from build123d import *

# Parameters (mm, degrees)
SKETCH1_W           = 57
SKETCH1_H           = 57
BOSS_EXTRUDE1_DEPTH = 113
SKETCH2_R           = 11
CUT_EXTRUDE1_DEPTH  = 103
SKETCH3_R           = 2.55
CUT_EXTRUDE2_DEPTH  = 120.97291361
FILLET2_R           = 3
SKETCH4_R           = 19
BOSS_EXTRUDE2_DEPTH = 1.6
FILLET4_R           = 3
SKETCH6_R           = 4
BOSS_EXTRUDE3_DEPTH = 24
SKETCH7_R           = 6
BOSS_EXTRUDE4_DEPTH = 2
CIRPATTERN4_COUNT   = 4
FILLET5_R           = 4
FILLET6_R           = 4


with BuildPart() as part:
    # Sketch1 → Boss-Extrude1 (new body)
    with BuildSketch(Plane.XY):
        Rectangle(SKETCH1_W, SKETCH1_H)
    extrude(amount=BOSS_EXTRUDE1_DEPTH)

    # Sketch2 → Cut-Extrude1 (cut)
    with BuildSketch(Plane(origin=(0, 0, 0), x_dir=(-1, 0, 0), z_dir=(0, 0, -1))):
        with Locations((-28.5, 28.5)):
            Circle(SKETCH2_R)
    cut_extrude1 = extrude(amount=-CUT_EXTRUDE1_DEPTH, mode=Mode.SUBTRACT)

    # Sketch3 → Cut-Extrude2 (cut, through all)
    with BuildSketch(Plane.XY.offset(113)):
        with Locations((-23.5, 23.5)):
            Circle(SKETCH3_R)
        with Locations((23.5, 23.5)):
            Circle(SKETCH3_R)
        with Locations((23.5, -23.5)):
            Circle(SKETCH3_R)
        with Locations((-23.5, -23.5)):
            Circle(SKETCH3_R)
    extrude(amount=-CUT_EXTRUDE2_DEPTH, mode=Mode.SUBTRACT)

    # Fillet2
    fillet2_edges = [part.edges().sort_by_distance(p)[0] for p in [
        (28.5, 28.5, 108),
    ]]
    fillet(fillet2_edges, radius=FILLET2_R)

    # Sketch4 → Boss-Extrude2 (add)
    with BuildSketch(Plane.XY.offset(113)):
        Circle(SKETCH4_R)
    extrude(amount=BOSS_EXTRUDE2_DEPTH)

    # Fillet4
    fillet4_edges = [part.edges().sort_by_distance(p)[0] for p in [
        (-28.5, 28.5, 56.5),
        (28.5, -28.5, 56.5),
        (-28.5, -28.5, 56.5),
    ]]
    fillet(fillet4_edges, radius=FILLET4_R)

    # Sketch6 → Boss-Extrude3 (add)
    with BuildSketch(Plane.XY.offset(114.6)):
        Circle(SKETCH6_R)
    extrude(amount=BOSS_EXTRUDE3_DEPTH)

    # Sketch7 → Boss-Extrude4 (add)
    with BuildSketch(Plane.ZY.offset(28.5)):
        with Locations(Location((12.240016964, 0, 0), (0, 0, 90))):
            Circle(SKETCH7_R)
    extrude(amount=BOSS_EXTRUDE4_DEPTH)

    # CirPattern4: Cut-Extrude1 ×4 about axis
    cirpattern4_axis = Axis((0, 0, 0), (0, 0, 1))
    for i in range(1, CIRPATTERN4_COUNT):
        add(cut_extrude1.rotate(cirpattern4_axis, i * 360 / CIRPATTERN4_COUNT), mode=Mode.SUBTRACT)

    # Fillet5
    fillet5_edges = [part.edges().sort_by_distance(p)[0] for p in [
        (-28.5, -17.5, 51.5),
        (-17.5, -28.5, 51.5),
        (17.5, -28.5, 51.5),
        (28.5, -17.5, 51.5),
        (28.5, 17.5, 51.5),
        (17.5, 28.5, 51.5),
        (-28.5, 17.5, 51.5),
        (-17.5, 28.5, 51.5),
    ]]
    fillet(fillet5_edges, radius=FILLET5_R)

    # Fillet6
    fillet6_edges = [part.edges().sort_by_distance(p)[0] for p in [
        (-28.5, 0, 0),
        (-20.721825407, 20.721825407, 0),
        (0, 28.5, 0),
        (20.721825407, 20.721825407, 0),
        (28.5, 0, 0),
        (20.721825407, -20.721825407, 0),
        (0, -28.5, 0),
        (-20.721825407, -20.721825407, 0),
        (27.683289703, -16.465287988, 0),
        (16.465287988, -27.683289703, 0),
        (-16.465287988, -27.683289703, 0),
        (-27.683289703, -16.465287988, 0),
        (27.683289703, 16.465287988, 0),
        (16.465287988, 27.683289703, 0),
        (-16.465287988, 27.683289703, 0),
        (-27.683289703, 16.465287988, 0),
    ]]
    fillet(fillet6_edges, radius=FILLET6_R)


solid = part.part
CAD build for the part. Positions are in the model's coordinates, mm. A direction names the side the tool comes from. Round coordinates to 2 decimals unless told otherwise and drop trailing zeros. Write each loop counter-clockwise with the first axis right and the second up, starting at its lowest first coordinate (ties: lowest second). Pieces come first, ordered by that corner, then holes.
(1) Probe line 1 along Y through (x, z) = (23.5, 109.75); line 2 along X through (y, z) = (-23, 107); line 3 along Z through (x, y) = (24.5, 0.5). List the from-to ranges inside material, lowest first.
(2) Drop flat-ended pins along their axis: P1, Ø3, axis at x = -23.5, y = -23.5, coming from the -Z side; P2, Ø6, axis at x = -22, y = 2, coming from the +Z side; P3, Ø16, axis at x = 24, y = 23.5, coming from the -Z side; P4, Ø6, axis at x = -4.5, y = -7, coming from the +Z side. Give the stop position or say it passes through.
(3) Slice it at B-B, the plane x = 0. Write the cut outline in (y, z), and give its area (3 significant figures).
(4) Slice it at A-A, the plane z = 42.5. Write the cut outline in (x, y), and give its area (3 significant figures).
(5) 3-axis set-ups, long thin cutter, end or side, ignore diameter. For faces 5 (the face through (-16.436, 27.705, 52.807)), 6 (the face through (26, 25, 103)), 7 (the face through (-0.867, -3.905, 126.432)): which of +Z, -Z, +X, -X, +Y, -Y reach the whole face in a straight line?
(6) Mould opens along X. For faces 1 (the face through (-25.4, 25.2, 108.1)), 2 (the face through (27.64, -27.6, 108.07)), 3 (the face through (21.476, -25.052, 108.07)), 4 (the face through (-0.197, -27.359, 1.203)) say: pulls with the +X half, pulls with the -X half, needs draft (parallel to the pull), parting line crosses it, or undercut.
From the geometry:
1. line 1: y = -28.5 to -26.05, -20.95 to 20.95, 26.05 to 28.5
1. line 2: x = -28.5 to -26, -21 to 21, 26 to 28.5
1. line 3: z = 0 to 113
2. P1: passes through
2. P2: stops at z = 113
2. P3: stops at z = 0.01
2. P4: stops at z = 114.6
3. outline: (-28.5, 4) arc R4 ccw to (-24.5, 0) - (24.5, 0) arc R4 ccw to (28.5, 4) - (28.5, 113) - (19, 113) - (19, 114.6) - (4, 114.6) - (4, 138.6) - (-4, 138.6) - (-4, 114.6) - (-19, 114.6) - (-19, 113) - (-28.5, 113) - close
3. area: 6,690 mm2
4. outline: (-28.5, -14.04) arc R4 ccw to (-25.57, -17.9) arc R11 cw to (-17.9, -25.57) arc R4 ccw to (-14.04, -28.5) - (14.04, -28.5) arc R4 ccw to (17.9, -25.57) arc R11 cw to (25.57, -17.9) arc R4 ccw to (28.5, -14.04) - (28.5, 14.04) arc R4 ccw to (25.57, 17.9) arc R11 cw to (17.9, 25.57) arc R4 ccw to (14.04, 28.5) - (-14.04, 28.5) arc R4 ccw to (-17.9, 25.57) arc R11 cw to (-25.57, 17.9) arc R4 ccw to (-28.5, 14.04) - close
4. area: 2,850 mm2
5. face 5: -Z, -X, +Y
5. face 6: -Z, +X, +Y
5. face 7: +Z
6. face 1: undercut
6. face 2: pulls with the +X half
6. face 3: undercut
6. face 4: needs draft
